Work out the finished part from the listing and answer in its coordinate system (mm). Coordinates: 2 decimals unless noted, no trailing zeros. Order: outer loops, then holes, each group sorted by start corner. A loop starts at its lowest first (then second) coordinate and runs counter-clockwise, first axis right, second up.
1. Flat-ended cylindrical pins translate along their axes: pin 1 Ø2 at (y, z) = (4, 6.5) entering from +X; pin 2 Ø8 at (y, z) = (11.5, 3) entering from +X; pin 3 Ø12 at (y, z) = (14.5, 19.5) entering from -X; pin 4 Ø2.5 at (x, z) = (-3, 2) entering from -Y. Find the tip coordinate at first contact, or state that the pin passes through.
2. The part is cut by section C-C, the plane z = 2.5. Give the vertices of the cut face in (x, y), then the cut area to 3 significant figures.
3. The part is cut by section A-A, the plane y = 0. Give the vertices of the cut face in (x, z), then the cut area to 3 significant figures.
4. Find the intervals of material crossed by probe 1 along X at (y, z) = (-5.5, 2.25); probe 2 along Y at (x, z) = (0, 6); probe 3 along Z at (x, y) = (-12.5, -8.5), in increasing order.
5. The part is cut by section D-D, the plane x = -12. Give the vertices of the cut face in (y, z), then the cut area to 3 significant figures.
6. Determine the mould class of faces 1 (the cylindrical face through (-1.08, -4.88, 8.87)), 2 (the flat face through (0, 0, 0)), 3 (the cylindrical face through (-15, 0, 2)) for opening direction Y: +Y half, -Y half, draft (parallel to the pull), parting line (faces both ways), or undercut.
```python
from build123d import *

# Parameters (mm, degrees)
SKETCH001_R       = 20
PAD001_DEPTH      = 5
CYLINDER012_R     = 5
CYLINDER012_DEPTH = 15


with BuildPart() as pad001:
    # Sketch001 → Pad001 (new body)
    with BuildSketch(Plane.XY):
        Circle(SKETCH001_R)
        with BuildLine():
            ThreePointArc((11.18034, -10), (15, 0), (11.18034, 10))
            Line((11.18034, 10), (11.18034, -10))
        make_face(mode=Mode.SUBTRACT)
        with BuildLine():
            ThreePointArc((-11.18034, 10), (-15, 0), (-11.18034, -10))
            Line((-11.18034, 10), (-11.18034, -10))
        make_face(mode=Mode.SUBTRACT)
        with BuildLine():
            ThreePointArc((10, 11.18034), (0, 15), (-10, 11.18034))
            Line((-10, 11.18034), (10, 11.18034))
        make_face(mode=Mode.SUBTRACT)
        with BuildLine():
            ThreePointArc((-10, -11.18034), (0, -15), (10, -11.18034))
            Line((-10, -11.18034), (10, -11.18034))
        make_face(mode=Mode.SUBTRACT)
    extrude(amount=PAD001_DEPTH)


with BuildPart() as sphere001:
    # Sphere001 → Sphere001 (revolve)
    with BuildSketch(Plane(origin=(0, 0, 17), x_dir=(1, 0, 0), z_dir=(0, -1, 0))):
        with BuildLine():
            ThreePointArc((0, -6.5), (6.5, 0), (0, 6.5))
            Line((0, 6.5), (0, -6.5))
        make_face()
    revolve(axis=Axis((0, 0, 17), (0, 0, 1)))


with BuildPart() as piezacirculo:
    # Cylinder012 → Cylinder012 (new body)
    with BuildSketch(Plane.XY):
        Circle(CYLINDER012_R)
    extrude(amount=CYLINDER012_DEPTH)

    # Fusion018: union Pad001, Sphere001
    add(pad001.part)
    add(sphere001.part)


solid = piezacirculo.part
```
Geometry says:
1. pin 1: stops at x = 4
1. pin 2: stops at x = 18.54
1. pin 3: passes through
1. pin 4: stops at y = -19.92
2. outline: circle Ø40 at (0, 0); hole (-11.18, -10) - (-11.18, 10) arc R15 ccw to start; hole (-10, -11.18) arc R15 ccw to (10, -11.18) - close; hole (-10, 11.18) - (10, 11.18) arc R15 ccw to start; hole (11.18, -10) arc R15 ccw to (11.18, 10) - close
2. area: 1,050 mm2
3. outline: (-20, 0) - (-15, 0) - (-15, 5) - (-20, 5) - close; (-11.18, 0) - (11.18, 0) - (11.18, 5) - (5, 5) - (5, 12.85) arc R6.5 ccw (long way) to (-5, 12.85) - (-5, 5) - (-11.18, 5) - close; (15, 0) - (20, 0) - (20, 5) - (15, 5) - close
3. area: 357 mm2
4. probe 1: x = -19.23 to -13.96, -11.18 to 11.18, 13.96 to 19.23
4. probe 2: y = -5 to 5
4. probe 3: z = 0 to 5
5. outline: (-16, 0) - (-9, 0) - (-9, 5) - (-16, 5) - close; (9, 0) - (16, 0) - (16, 5) - (9, 5) - close
5. area: 70.0 mm2
6. face 1: parting line
6. face 2: draft
6. face 3: undercut
